Source: CAD feature listing. Evaluate the final solid. Frame: model axes, mm. Face numbers are marked on the shaded views. A direction names the side the tool comes from. Give positions to 0.01 mm unless a question says otherwise; leave off trailing zeros. Write item = value, one per line.
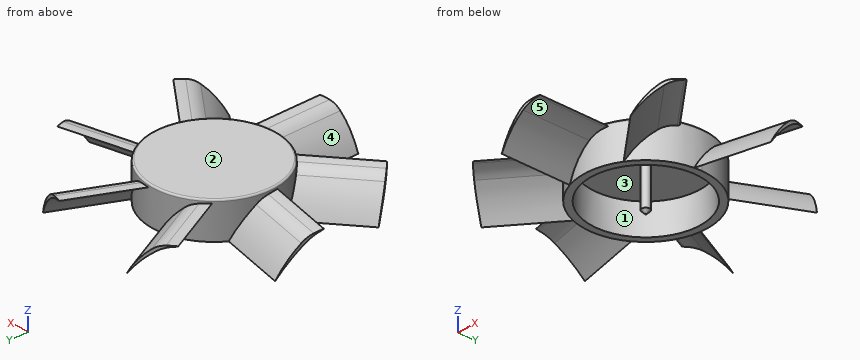
from build123d import *

# Parameters (mm, degrees)
SKETCH_1_R               = 11
EXTRUDE_1_DEPTH          = 6.5
SKETCH_2_R               = 9.75
CUT_EXTRUDE_1_DEPTH      = 5.5
SKETCH_3_R               = 0.7
EXTRUDE_2_DEPTH          = 7.5
CHAMFER_1_SIZE           = 0.6
EXTRUDE_START            = -10
EXTRUDE_3_DEPTH          = 23
PATTERN_CIRCULAR_1_COUNT = 7
FILLET_1_R               = 0.3
SKETCH_5_OUTSIDE_W       = 86.532
SKETCH_5_OUTSIDE_H       = 84.877
SKETCH_5_OUTSIDE_R       = 23
CUT_EXTRUDE_2_DEPTH      = 23


with BuildPart() as part:
    # Sketch 1 → Extrude 1 (new body)
    with BuildSketch(Plane.XY):
        Circle(SKETCH_1_R)
    extrude(amount=EXTRUDE_1_DEPTH)

    # Sketch 2 → Cut-Extrude 1 (cut)
    with BuildSketch(Plane(origin=(0, 0, 0), x_dir=(-1, 0, 0), z_dir=(0, 0, -1))):
        Circle(SKETCH_2_R)
    extrude(amount=-CUT_EXTRUDE_1_DEPTH, mode=Mode.SUBTRACT)

    # Sketch 3 → Extrude 2 (add)
    with BuildSketch(Plane(origin=(0, 0, 5.5), x_dir=(-1, 0, 0), z_dir=(0, 0, -1))):
        Circle(SKETCH_3_R)
    extrude(amount=EXTRUDE_2_DEPTH)

    # Chamfer 1
    chamfer_1_edges = [part.edges().sort_by_distance(p)[0] for p in [
        (0.7, 0, -2),
    ]]
    chamfer(chamfer_1_edges, length=CHAMFER_1_SIZE)

    # Sketch 4 → Extrude 3 (add)
    with BuildSketch(Plane(origin=(0, 0, 0), x_dir=(1, 0, 0), z_dir=(0, 1, 0)).offset(EXTRUDE_START)):
        with BuildLine():
            ThreePointArc((3.75, -5.9), (2.910954768, -5.877455841), (2.076425924, -5.787640746))
            ThreePointArc((2.076425924, -5.787640746), (1.016898237, -5.476222818), (0.082906283, -4.886952865))
            ThreePointArc((0.082906283, -4.886952865), (-2.084101368, -2.63998988), (-3.75, 0))
            ThreePointArc((-3.75, 0), (-1.712075741, -2.552424329), (0.739315837, -4.710822941))
            ThreePointArc((0.739315837, -4.710822941), (2.002660979, -5.416468702), (3.40130611, -5.787640746))
            ThreePointArc((3.40130611, -5.787640746), (3.575082247, -5.845591808), (3.75, -5.9))
        make_face()
    extrude_3 = extrude(amount=-EXTRUDE_3_DEPTH)

    # Pattern Circular 1: Extrude 3 ×7 about axis
    pattern_circular_1_axis = Axis((0, 0, 0), (0, 0, 1))
    for i in range(1, PATTERN_CIRCULAR_1_COUNT):
        add(extrude_3.rotate(pattern_circular_1_axis, i * 360 / PATTERN_CIRCULAR_1_COUNT))

    # Fillet 1
    fillet_1_edges = [part.edges().sort_by_distance(p)[0] for p in [
        (-11, 0, 6.5),
    ]]
    fillet(fillet_1_edges, radius=FILLET_1_R)

    # Sketch 5 outside → Cut-Extrude 2 (cut)
    with BuildSketch(Plane.XY.offset(6.5)):
        with Locations((0, -0.8205)):
            Rectangle(SKETCH_5_OUTSIDE_W, SKETCH_5_OUTSIDE_H)
        Circle(SKETCH_5_OUTSIDE_R, mode=Mode.SUBTRACT)
    extrude(amount=-CUT_EXTRUDE_2_DEPTH, mode=Mode.SUBTRACT)


solid = part.part
(1) First-contact query: pin 1 (1 mm diameter, centred on x = 12, z = -1, fed in from -Y); pin 2 (12 mm diameter, centred on x = 8, y = -1.5, fed in from -Z); pin 3 (5 mm diameter, centred on y = -11.5, z = 3.5, fed in from -X); pin 4 (6.5 mm diameter, centred on x = 1, y = 1.5, fed in from -Z). Flat tips, straight axial feed; report the tip coordinate or a pass-through.
Values follow:
pin_1 = through
pin_2 = 0
pin_3 = -19.8
pin_4 = -2
(2) Material intervals for line 1 (Y direction, x = 0, z = 4.2); line 2 (Y direction, x = 0, z = 2.65); line 3 (Y direction, x = -14, z = 4.5), sorted ascending.
Values follow:
line_1 = -23 to -9.75, -0.7 to 0.7, 9.75 to 11
line_2 = -11 to -9.75, -0.7 to 0.7, 9.75 to 11
line_3 = -11.75 to -10.71, 2.73 to 3.56
(3) Access query for the marked faces 4 and 5. Directions: +Z, -Z, +X, -X, +Y, -Y. A direction counts if a zero-diameter tool reaches every point of the face in a straight line with its end or side. Return the directions, or none.
Values follow:
face_4 = +Z, -Y
face_5 = -Z, -Y
(4) Pull-direction query (Y, two-part tool) for the marked faces 1, 2 and 3; classes: pulls with the +Y half, pulls with the -Y half, needs draft (parallel to the pull), parting line crosses it, or undercut.
Values follow:
face_1 = undercut
face_2 = needs draft
face_3 = undercut
